Can you work these out from the model? Positions are in its coordinate system, mm. Face numbers are marked on the shaded views. A direction names the side the tool comes from. Round coordinates to 2 decimals unless told otherwise and drop trailing zeros. Write each loop counter-clockwise with the first axis right and the second up, starting at its lowest first coordinate (ties: lowest second). Pieces come first, ordered by that corner, then holes.
Q1. We'd pull the mould along Z, two halves only. Please class the marked faces 1, 2 and 3: +Z half, -Z half, draft (parallel to the pull), parting line (faces both ways), or undercut.
Q2. If we section it at D-D (x = -45.5): Please give me the cut outline in (y, z).
Q3. If we section it at C-C (y = 6.75): Give the number of separate pieces and of enclosed holes in the cut face, plus the area to 3 significant figures.
Q4. Please list where these lines run through material, in increasing order: line 1 along X through (y, z) = (10.5, 0) (3 decimals); line 2 along X through (y, z) = (7, -5) (3 decimals); line 3 along Z through (x, y) = (-8, 8.5).
Q5. If we section it at A-A (x = 49.5): Please give me the cut outline in (y, z).
Q6. If we section it at B-B (z = 0): Please give me the cut outline in (x, y) (3 decimals).
Q7. For the marked faces 4 and 5, which set-ups out of +Z, -Z, +X, -X, +Y, -Y let a thin tool reach every point of the face, with its end or its side?
Q8. I'm going to push flat-ended pins straight in: pin 1 Ø1 at (x, z) = (-52, -34) entering from +Y; pin 2 Ø7 at (x, z) = (49, -23) entering from +Y. Where does each tip first touch, or does it pass through?
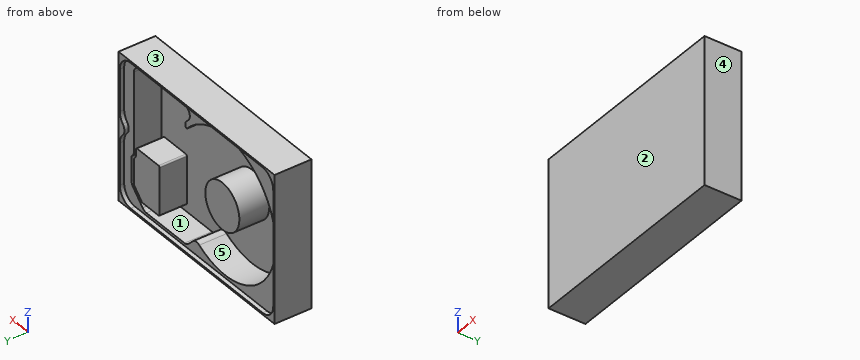
from build123d import *

# Parameters (mm, degrees)
SKETCH1_W           = 146.65
SKETCH1_H           = 101.42
BOSS_EXTRUDE1_DEPTH = 25.4
CUT_EXTRUDE1_DEPTH  = 3
FILLET1_R           = 10
SKETCH3_R           = 47.7
CUT_EXTRUDE2_DEPTH  = 18.8
FILLET2_R           = 5
SKETCH4_R           = 16
BOSS_EXTRUDE2_DEPTH = 20.6
BOSS_EXTRUDE3_DEPTH = 18.8
FILLET4_R           = 1
FILLET5_R           = 5


with BuildPart() as part:
    # Sketch1 → Boss-Extrude1 (new body)
    with BuildSketch(Plane(origin=(0, 0, 0), x_dir=(1, 0, 0), z_dir=(0, 1, 0))):
        Rectangle(SKETCH1_W, SKETCH1_H)
    extrude(amount=BOSS_EXTRUDE1_DEPTH)

    # Sketch2 → Cut-Extrude1 (cut)
    with BuildSketch(Plane(origin=(0, 25.4, 0), x_dir=(1, 0, 0), z_dir=(0, 1, 0))):
        with BuildLine():
            Line((-72.125, 49.51), (-72.125, -49.51))
            Line((-72.125, -49.51), (72.125, -49.51))
            Line((72.125, -49.51), (72.125, -5.36749476))
            ThreePointArc((72.125, -5.36749476), (67.825, 0), (72.125, 5.36749476))
            Line((72.125, 5.36749476), (72.125, 49.51))
            Line((72.125, 49.51), (-72.125, 49.51))
        make_face()
    extrude(amount=-CUT_EXTRUDE1_DEPTH, mode=Mode.SUBTRACT)

    # Fillet1
    fillet1_edges = [part.edges().sort_by_distance(p)[0] for p in [
        (72.125, 23.9, -5.36749476),
        (72.125, 23.9, 5.36749476),
        (72.125, 23.9, 49.51),
        (-72.125, 23.9, 49.51),
        (-72.125, 23.9, -49.51),
        (72.125, 23.9, -49.51),
    ]]
    fillet(fillet1_edges, radius=FILLET1_R)

    # Sketch3 → Cut-Extrude2 (cut)
    with BuildSketch(Plane(origin=(0, 22.4, 0), x_dir=(1, 0, 0), z_dir=(0, 1, 0))):
        with BuildLine():
            Line((3.325, -46.51), (62.925, -46.51))
            Line((62.925, -46.51), (62.925, 14.7))
            Line((62.925, 14.7), (65.225, 17))
            Line((65.225, 17), (65.225, 35.8))
            Line((65.225, 35.8), (53.325, 47.7))
            Line((53.325, 47.7), (13.325, 47.7))
            Line((13.325, 47.7), (4.71750668, 39.09250668))
            ThreePointArc((4.71750668, 39.09250668), (19.687781047, 22.040070682), (25.085, 0))
            ThreePointArc((25.085, 0), (22.099291128, -16.610905119), (13.515936315, -31.142341611))
            ThreePointArc((13.515936315, -31.142341611), (14.64327542, -33.663677787), (13.61, -36.225))
            Line((13.61, -36.225), (3.325, -46.51))
        make_face()
        with Locations((-22.615, 0)):
            Circle(SKETCH3_R)
    extrude(amount=-CUT_EXTRUDE2_DEPTH, mode=Mode.SUBTRACT)

    # Fillet2
    fillet2_edges = [part.edges().sort_by_distance(p)[0] for p in [
        (4.71750668, 13, -39.09250668),
        (13.325, 13, -47.7),
        (53.325, 13, -47.7),
        (65.225, 13, -35.8),
        (62.925, 13, -14.7),
        (62.925, 13, 46.51),
        (3.325, 13, 46.51),
    ]]
    fillet(fillet2_edges, radius=FILLET2_R)

    # Sketch4 → Boss-Extrude2 (add)
    with BuildSketch(Plane(origin=(0, 3.6, 0), x_dir=(1, 0, 0), z_dir=(0, 1, 0))):
        with Locations(Location((-22.615, 0, 0), (0, 0, 90))):
            Circle(SKETCH4_R)
    extrude(amount=BOSS_EXTRUDE2_DEPTH)

    # Sketch5 → Boss-Extrude3 (add)
    with BuildSketch(Plane(origin=(0, 3.6, 0), x_dir=(1, 0, 0), z_dir=(0, 1, 0))):
        Polygon((38.825, 42.9), (55.296572875, 42.9), (62.725, 35.471572875), (62.725, 17), (60.925, 15.2), (60.925, 8.9), (38.825, 8.9), align=None)
    extrude(amount=BOSS_EXTRUDE3_DEPTH)

    # Fillet4
    fillet4_edges = [part.edges().sort_by_distance(p)[0] for p in [
        (38.825, 13, -42.9),
        (38.825, 13, -8.9),
        (60.925, 13, -8.9),
        (62.725, 13, -17),
        (62.725, 13, -35.471572875),
        (55.296572875, 13, -42.9),
    ]]
    fillet(fillet4_edges, radius=FILLET4_R)

    # Fillet5
    fillet5_edges = [part.edges().sort_by_distance(p)[0] for p in [
        (60.925, 13, -15.2),
    ]]
    fillet(fillet5_edges, radius=FILLET5_R)


solid = part.part
A:
1. face 1: undercut
1. face 2: draft
1. face 3: +Z half
2. outline: (0, -50.71) - (25.4, -50.71) - (25.4, -49.51) - (22.4, -49.51) - (22.4, -41.85) - (3.6, -41.85) - (3.6, 41.85) - (22.4, 41.85) - (22.4, 49.51) - (25.4, 49.51) - (25.4, 50.71) - (0, 50.71) - close
3. separate pieces: 3
3. enclosed holes: 1
3. area: 5,050 mm2
4. line 1: x = -73.325 to -70.315, -38.615 to -6.615, 62.925 to 73.325
4. line 2: x = -73.325 to -70.052, -37.814 to -7.416, 62.925 to 73.325
4. line 3: z = -50.71 to -45.41, -6.51 to 6.51, 45.41 to 50.71
5. outline: (0, -50.71) - (25.4, -50.71) - (25.4, -49.51) - (22.4, -49.51) - (22.4, -47.7) - (3.6, -47.7) - (3.6, -42.9) - (22.4, -42.9) - (22.4, -8.9) - (3.6, -8.9) - (3.6, 46.51) - (22.4, 46.51) - (22.4, 49.51) - (25.4, 49.51) - (25.4, 50.71) - (0, 50.71) - close
6. outline: (-73.325, 0) - (73.325, 0) - (73.325, 25.4) - (67.825, 25.4) - (67.825, 22.4) - (62.925, 22.4) - (62.925, 3.6) - (-6.615, 3.6) - (-6.615, 24.2) - (-38.615, 24.2) - (-38.615, 3.6) - (-70.315, 3.6) - (-70.315, 22.4) - (-72.125, 22.4) - (-72.125, 25.4) - (-73.325, 25.4) - close
7. face 4: +Z, -Z, +X, +Y, -Y
7. face 5: +Y
8. pin 1: stops at y = 3.6
8. pin 2: stops at y = 22.4
